For this review, take the finished solid that the model builds, in its own axes (mm). Give positions to 0.01 mm unless a question says otherwise; leave off trailing zeros. Loops run counter-clockwise (first coordinate to the right, second up) from the corner with the lowest first, then second, coordinate; pieces in that order, holes last.
```python
from build123d import *

# Parameters (mm, degrees)
SKETCH_1_R      = 1.5
EXTRUDE_1_DEPTH = 2


with BuildPart() as part:
    # 草图1 → 凸台-拉伸1 (new body)
    with BuildSketch(Plane.XY):
        Polygon((3, 3.164176285), (0, 32), (-3, 3.164176285), (-3, -13.164176285), (3, -13.164176285), align=None)
        Circle(SKETCH_1_R, mode=Mode.SUBTRACT)
        with Locations((0, -10)):
            Circle(SKETCH_1_R, mode=Mode.SUBTRACT)
    extrude(amount=EXTRUDE_1_DEPTH)


solid = part.part
```
Item 1: The part is to be moulded in two halves that separate along Y. For faces 1 (the cylindrical face through (-1.5, 0.07, 0.99)), 2 (the flat face through (0, -13.164, 1)), 3 (the flat face through (0, 5, 0)), say which applies: released by +Y, released by -Y, zero draft, split by the parting line, or undercut.
Answer:
face 1: undercut
face 2: released by -Y
face 3: zero draft
Item 2: Take a section at B-B on x = -0.6. Give the boundary of the cut face in (y, z), and give its area (3 significant figures).
Answer:
outline: (-13.16, 0) - (-11.37, 0) - (-11.37, 2) - (-13.16, 2) - close; (-8.63, 0) - (-1.37, 0) - (-1.37, 2) - (-8.63, 2) - close; (1.37, 0) - (26.23, 0) - (26.23, 2) - (1.37, 2) - close
area: 67.8 mm2
Item 3: Take a section at D-D on x = -2.35. Give the boundary of the cut face in (y, z).
Answer:
outline: (-13.16, 0) - (9.41, 0) - (9.41, 2) - (-13.16, 2) - close
Item 4: Take a section at C-C on z = 0.55. Give the boundary of the cut face in (x, y), and give its area (3 significant figures).
Answer:
outline: (-3, -13.16) - (3, -13.16) - (3, 3.16) - (0, 32) - (-3, 3.16) - close; hole circle Ø3 at (0, -10); hole circle Ø3 at (0, 0)
area: 170 mm2
Item 5: Take a section at A-A on y = 0. Give the boundary of the cut face in (x, z).
Answer:
outline: (-3, 0) - (-1.5, 0) - (-1.5, 2) - (-3, 2) - close; (1.5, 0) - (3, 0) - (3, 2) - (1.5, 2) - close
Item 6: For L1, parallel to X at y = 16, z = 0.3; L2, parallel to X at y = 24, z = 0.9, list the stretches that pass through material, from the lowest coordinate up.
Answer:
L1: x = -1.66 to 1.66
L2: x = -0.83 to 0.83
